The model under review builds one solid part; all positions refer to its coordinate system, in mm. A direction names the side the tool comes from. Round coordinates to 2 decimals unless told otherwise and drop trailing zeros. Write each question's results on one line, items separated by ' | '.
```python
from build123d import *

# Parameters (mm, degrees)
SKETCH1_W                        = 234.95
SKETCH1_H                        = 25.4
BOSS_EXTRUDE1_DEPTH              = 9.525
F_8_CLEARANCE_HOLE1_D            = 4.4958
F_8_CLEARANCE_HOLE1_DEPTH        = 25.4
F_8_CLEARANCE_HOLE1_TIP          = 1.350674586
F_8_CLEARANCE_HOLE2_D            = 4.4958
F_8_CLEARANCE_HOLE2_DEPTH        = 19.05
F_8_CLEARANCE_HOLE2_TIP          = 1.350674586
F_4_CLEARANCE_HOLE3_D            = 3.2639
F_4_CLEARANCE_HOLE2_D            = 3.2639
F_4_CLEARANCE_HOLE2_DEPTH        = 9.525
F_1_8_0_125_DIAMETER_HOLE1_D     = 3.175
F_1_8_0_125_DIAMETER_HOLE1_DEPTH = 9.525
SKETCH18_W                       = 15.875
SKETCH18_H                       = 25.4
SKETCH18_R                       = 2.2479
CUT_EXTRUDE1_DEPTH               = 1.27
CHAMFER1_SIZE                    = 0.508


with BuildPart() as part:
    # Sketch1 → Boss-Extrude1 (new body)
    with BuildSketch(Plane.XY):
        with Locations((-117.475, 12.7)):
            Rectangle(SKETCH1_W, SKETCH1_H)
    extrude(amount=BOSS_EXTRUDE1_DEPTH)

    # #8 Clearance Hole1
    with Locations(Plane.XY.offset(9.525)):
        with Locations((-7.9375, 6.35), (-7.9375, 19.05)):
            Hole(F_8_CLEARANCE_HOLE1_D / 2, depth=F_8_CLEARANCE_HOLE1_DEPTH)
            with Locations((0, 0, -(F_8_CLEARANCE_HOLE1_DEPTH + F_8_CLEARANCE_HOLE1_TIP / 2))):  # 118° drill point
                Cone(0, F_8_CLEARANCE_HOLE1_D / 2, F_8_CLEARANCE_HOLE1_TIP, mode=Mode.SUBTRACT)

    # #8 Clearance Hole2
    with Locations(Plane.XY.offset(9.525)):
        with Locations((-147.6375, 12.7)):
            Hole(F_8_CLEARANCE_HOLE2_D / 2, depth=F_8_CLEARANCE_HOLE2_DEPTH)
            with Locations((0, 0, -(F_8_CLEARANCE_HOLE2_DEPTH + F_8_CLEARANCE_HOLE2_TIP / 2))):  # 118° drill point
                Cone(0, F_8_CLEARANCE_HOLE2_D / 2, F_8_CLEARANCE_HOLE2_TIP, mode=Mode.SUBTRACT)

    # #4 Clearance Hole3 (through all)
    with Locations(Plane(origin=(0, 0, 0), x_dir=(-1, 0, 0), z_dir=(0, 0, -1))):
        with Locations((103.1875, 12.7), (52.3875, 12.7)):
            Hole(F_4_CLEARANCE_HOLE3_D / 2)

    # #4 Clearance Hole2
    with Locations(Plane.XY.offset(9.525)):
        with Locations((-223.8375, 12.7), (-198.4375, 12.7)):
            Hole(F_4_CLEARANCE_HOLE2_D / 2, depth=F_4_CLEARANCE_HOLE2_DEPTH)

    # 1/8 (0.125) Diameter Hole1
    with Locations(Plane.XY.offset(9.525)):
        with Locations((-19.05, 4.7625), (-85.725, 20.6375), (-128.5875, 4.7625)):
            Hole(F_1_8_0_125_DIAMETER_HOLE1_D / 2, depth=F_1_8_0_125_DIAMETER_HOLE1_DEPTH)

    # Sketch18 → Cut-Extrude1 (cut)
    with BuildSketch(Plane(origin=(0, 0, 0), x_dir=(-1, 0, 0), z_dir=(0, 0, -1))):
        with Locations((7.9375, 12.7)):
            Rectangle(SKETCH18_W, SKETCH18_H)
        with Locations((7.9375, 6.35)):
            Circle(SKETCH18_R, mode=Mode.SUBTRACT)
    extrude(amount=-CUT_EXTRUDE1_DEPTH, mode=Mode.SUBTRACT)

    # Chamfer1
    chamfer1_edges = [part.edges().sort_by_distance(p)[0] for p in [
        (-234.95, 12.7, 9.525),
        (0, 12.7, 9.525),
        (-234.95, 12.7, 0),
        (0, 0, 5.3975),
        (-234.95, 0, 4.7625),
        (-234.95, 25.4, 4.7625),
        (0, 25.4, 5.3975),
        (0, 12.7, 1.27),
    ]]
    chamfer(chamfer1_edges, length=CHAMFER1_SIZE)


solid = part.part
```
Q1. For probe 1 along X at (y, z) = (5.75, 4.25); probe 2 along Y at (x, z) = (-19.05, 6.5) (3 decimals); probe 3 along X at (y, z) = (5.25, 5.25), list the stretches that pass through material, from the lowest coordinate up.
Evaluation:
probe 1: x = -234.95 to -129.83, -127.34 to -20.29, -17.81 to -10.1, -5.77 to 0 | probe 2: y = 0 to 3.175, 6.35 to 25.4 | probe 3: x = -234.95 to -130.1, -127.08 to -20.56, -17.54 to -9.9, -5.98 to 0
Q2. Tool access review of faces 1 (the flat face through (-8, 13, 1.27)), 2 (the cylindrical face through (-10.08, 7.03, 5.34)): name each direction out of +Z, -Z, +X, -X, +Y, -Y from which nothing blocks a thin tool from reaching the whole face with its end or side.
Evaluation:
face 1: -Z, +X, +Y, -Y | face 2: +Z, -Z
Q3. Insertion check: P1, Ø7, axis at x = -7.94, y = 6.35, coming from the +Z side (3 decimals); P2, Ø7.5, axis at x = -5.5, y = 7.5, coming from the -Z side; P3, Ø1.4, axis at y = 11, z = 0.5, coming from the +X side (3 decimals). Each pin has a flat end and moves straight along its axis. Give the tip position at first contact, or say it passes through.
Evaluation:
P1: stops at z = 9.525 | P2: stops at z = 1.27 | P3: stops at x = -15.875
Q4. The part is to be moulded in two halves that separate along Y. For faces 3 (the cylindrical face through (-10.08, 19.73, 5.34)), 4 (the flat face through (-119, 0, 5)), 5 (the flat face through (-119, 13, 9.525)), say which applies: released by +Y, released by -Y, zero draft, split by the parting line, or undercut.
Evaluation:
face 3: undercut | face 4: released by -Y | face 5: zero draft
Q5. We need section A-A (z = 5.25). State how many separate pieces and enclosed holes the cut face has, plus the area to 3 significant figures.
Evaluation:
separate pieces: 1 | enclosed holes: 10 | area: 5,860 mm^2
